Autodesk Inventor part; units mm, degrees
ref_plane "YZ Plane" through (0, 0, 0) normal (1, 0, 0) x (0, 1, 0)
ref_plane "XZ Plane" through (0, 0, 0) normal (0, 1, 0) x (-1, 0, 0)
ref_plane "XY Plane" through (0, 0, 0) normal (0, 0, 1) x (1, 0, 0)
sketch "Skizze1" plane through (0, 0, 0) normal (0, 0, 1) x (1, 0, 0)
  line L0 (2.5, 0) -> (30.5, 0)
  line L1 (33, 2.5) -> (33, 2.5)
  line L2 (30.5, 5) -> (2.5, 5)
  line L3 (0, 2.5) -> (0, 2.5)
  arc A0 (2.5, 5) -> (0, 2.5) centre (2.5, 2.5) ccw
  arc A1 (0, 2.5) -> (2.5, 0) centre (2.5, 2.5) ccw
  arc A2 (33, 2.5) -> (30.5, 5) centre (30.5, 2.5) ccw
  arc A3 (30.5, 0) -> (33, 2.5) centre (30.5, 2.5) ccw
  point P0 (0, 0)
  point P1 (33, 5)
  point P2 (0, 5)
  dimension "d0" = 33
  dimension "d9" = 2.5
  dimension "d19" = 5
extrude "Extrusion2" add sketch "Skizze1" along normal blind 4
sketch "Skizze2" plane through (0, 0, 4) normal (0, 0, 1) x (1, 0, 0)
  arc A0 (2.5, 5) -> (2.5, 0) centre (2.5, 2.5) ccw
  circle A1 centre (2.5, 2.5) radius 0.75
  arc A2 (30.5, 0) -> (30.5, 5) centre (30.5, 2.5) ccw
  circle A3 centre (30.5, 2.5) radius 0.75
  point P0 (0, 0)
  dimension "d15" = 1.5
  dimension "d16" = 1.5
extrude "Extrusion3" cut sketch "Skizze2" against normal blind 4
properties part number "Klemme_Hebel_Entstück"
Source: CAD feature listing. Evaluate the final solid. Frame: model axes, mm. Round coordinates to 2 decimals unless told otherwise and drop trailing zeros. Loops run counter-clockwise (first coordinate to the right, second up) from the corner with the lowest first, then second, coordinate; pieces in that order, holes last.
Q1. Ray query, line 1 (Y direction, x = 2.5, z = 2.4); line 2 (X direction, y = 2.9, z = 3.3); line 3 (Y direction, x = 3, z = 2.35). Return the intervals inside material, ascending.
Q2. Mould query, pull axis Y, two halves, no side actions, for faces 1 (the face through (3.19, 2.21, 2.03)), 2 (the face through (16, 0, 2)), 3 (the face through (33, 2.6, 2)), 4 (the face through (31.215, 2.725, 2.028)). Classes: pulls with the +Y half, pulls with the -Y half, needs draft (parallel to the pull), parting line crosses it, or undercut.
Q3. Section B-B, the plane z = 1.05. Return loops of the section in (x, y), plus the area to 3 significant figures.
Q4. Section C-C, the plane y = 4.55. Return loops of the section in (x, z), plus the area to 3 significant figures.
Q5. First-contact query: P1, Ø2, axis at x = 30.5, y = 2.5, coming from the -Z side; P2, Ø2, axis at y = 4.5, z = 2, coming from the -X side. Flat tips, straight axial feed; report the tip coordinate or a pass-through.
Q6. Section A-A, the plane y = 2.5. Return loops of the section in (x, z).
Solutions:
1. line 1: y = 0 to 1.75, 3.25 to 5
1. line 2: x = 0.03 to 1.87, 3.13 to 29.87, 31.13 to 32.97
1. line 3: y = 0 to 1.94, 3.06 to 5
2. face 1: undercut
2. face 2: pulls with the -Y half
2. face 3: parting line crosses it
2. face 4: undercut
3. outline: (2.5, 0) - (30.5, 0) arc R2.5 ccw to (30.5, 5) - (2.5, 5) arc R2.5 ccw to start; hole circle Ø1.5 at (2.5, 2.5); hole circle Ø1.5 at (30.5, 2.5)
3. area: 156 mm2
4. outline: (1.07, 0) - (31.93, 0) - (31.93, 4) - (1.07, 4) - close
4. area: 123 mm2
5. P1: stops at z = 0
5. P2: stops at x = 0.21
6. outline: (0, 0) - (1.75, 0) - (1.75, 4) - (0, 4) - close; (3.25, 0) - (29.75, 0) - (29.75, 4) - (3.25, 4) - close; (31.25, 0) - (33, 0) - (33, 4) - (31.25, 4) - close
